```python
from build123d import *

# Parameters (mm, degrees)
SKETCH_1_R               = 72.2
EXTRUDE_1_DEPTH          = 9
CUT_EXTRUDE_START        = -9
CUT_EXTRUDE_2_DEPTH      = 9
SKETCH_3_R               = 47
CUT_EXTRUDE_3_DEPTH      = 3
CUT_EXTRUDE_START_2      = -3
SKETCH_4_R               = 47
CUT_EXTRUDE_4_DEPTH      = 3
SKETCH_6_R               = 2
CUT_EXTRUDE_6_DEPTH      = 3
PATTERN_CIRCULAR_1_COUNT = 14
SKETCH_5_R               = 13
SKETCH_5_R_2             = 2.5
SKETCH_5_R_3             = 10.5
CUT_EXTRUDE_7_DEPTH      = 102.792337629


with BuildPart() as part:
    # 草图1 → 凸台-拉伸1 (new body)
    with BuildSketch(Plane.XY):
        Circle(SKETCH_1_R)
    extrude(amount=EXTRUDE_1_DEPTH)

    # 草图2 → 切除-拉伸2 (cut)
    with BuildSketch(Plane.XY.offset(9).offset(CUT_EXTRUDE_START)):
        with BuildLine():
            Line((-10, 71.504125755), (-10, 59.666070761))
            ThreePointArc((-10, 59.666070761), (-9.316897592, 58.160819708), (-7.734219269, 57.683809273))
            ThreePointArc((-7.734219269, 57.683809273), (0, 58.2), (7.734219269, 57.683809273))
            ThreePointArc((7.734219269, 57.683809273), (9.316897592, 58.160819708), (10, 59.666070761))
            Line((10, 59.666070761), (10, 71.504125755))
            ThreePointArc((10, 71.504125755), (0, 72.2), (-10, 71.504125755))
        make_face()
        with BuildLine():
            Line((22.014788766, 68.761828623), (16.878449201, 58.096109616))
            ThreePointArc((16.878449201, 58.096109616), (16.840799249, 56.443538253), (18.059776075, 55.327068313))
            ThreePointArc((18.059776075, 55.327068313), (25.252033617, 52.436388112), (31.996357633, 48.615564362))
            ThreePointArc((31.996357633, 48.615564362), (33.629268601, 48.358637524), (34.897826559, 49.418434834))
            Line((34.897826559, 49.418434834), (40.034166124, 60.084153841))
            ThreePointArc((40.034166124, 60.084153841), (31.326405964, 65.049952263), (22.014788766, 68.761828623))
        make_face()
        with BuildLine():
            Line((49.669278623, 52.400408024), (40.413914537, 45.019501461))
            ThreePointArc((40.413914537, 45.019501461), (39.66296926, 43.546921812), (40.276811279, 42.012122931))
            ThreePointArc((40.276811279, 42.012122931), (45.50259228, 36.287106468), (49.921224958, 29.918410697))
            ThreePointArc((49.921224958, 29.918410697), (51.280950528, 28.978434099), (52.883710574, 29.382871811))
            Line((52.883710574, 29.382871811), (62.13907466, 36.763778374))
            ThreePointArc((62.13907466, 36.763778374), (56.448233034, 45.015963694), (49.669278623, 52.400408024))
        make_face()
        with BuildLine():
            Line((67.486158695, 25.660443967), (55.944908455, 23.026228913))
            ThreePointArc((55.944908455, 23.026228913), (54.629401775, 22.025303439), (54.516530046, 20.376161358))
            ThreePointArc((54.516530046, 20.376161358), (56.740804489, 12.950718356), (57.958581437, 5.295548869))
            ThreePointArc((57.958581437, 5.295548869), (58.775811283, 3.858696403), (60.395327134, 3.527670669))
            Line((60.395327134, 3.527670669), (71.936577374, 6.161885723))
            ThreePointArc((71.936577374, 6.161885723), (70.38979526, 16.066011432), (67.486158695, 25.660443967))
        make_face()
        with BuildLine():
            Line((71.936577374, -6.161885723), (60.395327134, -3.527670669))
            ThreePointArc((60.395327134, -3.527670669), (58.775811283, -3.858696403), (57.958581437, -5.295548869))
            ThreePointArc((57.958581437, -5.295548869), (56.740804489, -12.950718356), (54.516530046, -20.376161358))
            ThreePointArc((54.516530046, -20.376161358), (54.629401775, -22.025303439), (55.944908455, -23.026228913))
            Line((55.944908455, -23.026228913), (67.486158695, -25.660443967))
            ThreePointArc((67.486158695, -25.660443967), (70.38979526, -16.066011432), (71.936577374, -6.161885723))
        make_face()
        with BuildLine():
            Line((62.13907466, -36.763778374), (52.883710574, -29.382871811))
            ThreePointArc((52.883710574, -29.382871811), (51.280950528, -28.978434099), (49.921224958, -29.918410697))
            ThreePointArc((49.921224958, -29.918410697), (45.50259228, -36.287106468), (40.276811279, -42.012122931))
            ThreePointArc((40.276811279, -42.012122931), (39.66296926, -43.546921812), (40.413914537, -45.019501461))
            Line((40.413914537, -45.019501461), (49.669278623, -52.400408024))
            ThreePointArc((49.669278623, -52.400408024), (56.448233034, -45.015963694), (62.13907466, -36.763778374))
        make_face()
        with BuildLine():
            Line((40.034166124, -60.084153841), (34.897826559, -49.418434834))
            ThreePointArc((34.897826559, -49.418434834), (33.629268601, -48.358637524), (31.996357633, -48.615564362))
            ThreePointArc((31.996357633, -48.615564362), (25.252033617, -52.436388112), (18.059776075, -55.327068313))
            ThreePointArc((18.059776075, -55.327068313), (16.840799249, -56.443538253), (16.878449201, -58.096109616))
            Line((16.878449201, -58.096109616), (22.014788766, -68.761828623))
            ThreePointArc((22.014788766, -68.761828623), (31.326405964, -65.049952263), (40.034166124, -60.084153841))
        make_face()
        with BuildLine():
            Line((10, -71.504125755), (10, -59.666070761))
            ThreePointArc((10, -59.666070761), (9.316897592, -58.160819708), (7.734219269, -57.683809273))
            ThreePointArc((7.734219269, -57.683809273), (0, -58.2), (-7.734219269, -57.683809273))
            ThreePointArc((-7.734219269, -57.683809273), (-9.316897592, -58.160819708), (-10, -59.666070761))
            Line((-10, -59.666070761), (-10, -71.504125755))
            ThreePointArc((-10, -71.504125755), (0, -72.2), (10, -71.504125755))
        make_face()
        with BuildLine():
            Line((-22.014788766, -68.761828623), (-16.878449201, -58.096109616))
            ThreePointArc((-16.878449201, -58.096109616), (-16.840799249, -56.443538253), (-18.059776075, -55.327068313))
            ThreePointArc((-18.059776075, -55.327068313), (-25.252033617, -52.436388112), (-31.996357633, -48.615564362))
            ThreePointArc((-31.996357633, -48.615564362), (-33.629268601, -48.358637524), (-34.897826559, -49.418434834))
            Line((-34.897826559, -49.418434834), (-40.034166124, -60.084153841))
            ThreePointArc((-40.034166124, -60.084153841), (-31.326405964, -65.049952263), (-22.014788766, -68.761828623))
        make_face()
        with BuildLine():
            Line((-49.669278623, -52.400408024), (-40.413914537, -45.019501461))
            ThreePointArc((-40.413914537, -45.019501461), (-39.66296926, -43.546921812), (-40.276811279, -42.012122931))
            ThreePointArc((-40.276811279, -42.012122931), (-45.50259228, -36.287106468), (-49.921224958, -29.918410697))
            ThreePointArc((-49.921224958, -29.918410697), (-51.280950528, -28.978434099), (-52.883710574, -29.382871811))
            Line((-52.883710574, -29.382871811), (-62.13907466, -36.763778374))
            ThreePointArc((-62.13907466, -36.763778374), (-56.448233034, -45.015963694), (-49.669278623, -52.400408024))
        make_face()
        with BuildLine():
            Line((-67.486158695, -25.660443967), (-55.944908455, -23.026228913))
            ThreePointArc((-55.944908455, -23.026228913), (-54.629401775, -22.025303439), (-54.516530046, -20.376161358))
            ThreePointArc((-54.516530046, -20.376161358), (-56.740804489, -12.950718356), (-57.958581437, -5.295548869))
            ThreePointArc((-57.958581437, -5.295548869), (-58.775811283, -3.858696403), (-60.395327134, -3.527670669))
            Line((-60.395327134, -3.527670669), (-71.936577374, -6.161885723))
            ThreePointArc((-71.936577374, -6.161885723), (-70.38979526, -16.066011432), (-67.486158695, -25.660443967))
        make_face()
        with BuildLine():
            Line((-71.936577374, 6.161885723), (-60.395327134, 3.527670669))
            ThreePointArc((-60.395327134, 3.527670669), (-58.775811283, 3.858696403), (-57.958581437, 5.295548869))
            ThreePointArc((-57.958581437, 5.295548869), (-56.740804489, 12.950718356), (-54.516530046, 20.376161358))
            ThreePointArc((-54.516530046, 20.376161358), (-54.629401775, 22.025303439), (-55.944908455, 23.026228913))
            Line((-55.944908455, 23.026228913), (-67.486158695, 25.660443967))
            ThreePointArc((-67.486158695, 25.660443967), (-70.38979526, 16.066011432), (-71.936577374, 6.161885723))
        make_face()
        with BuildLine():
            Line((-62.13907466, 36.763778374), (-52.883710574, 29.382871811))
            ThreePointArc((-52.883710574, 29.382871811), (-51.280950528, 28.978434099), (-49.921224958, 29.918410697))
            ThreePointArc((-49.921224958, 29.918410697), (-45.50259228, 36.287106468), (-40.276811279, 42.012122931))
            ThreePointArc((-40.276811279, 42.012122931), (-39.66296926, 43.546921812), (-40.413914537, 45.019501461))
            Line((-40.413914537, 45.019501461), (-49.669278623, 52.400408024))
            ThreePointArc((-49.669278623, 52.400408024), (-56.448233034, 45.015963694), (-62.13907466, 36.763778374))
        make_face()
        with BuildLine():
            Line((-40.034166124, 60.084153841), (-34.897826559, 49.418434834))
            ThreePointArc((-34.897826559, 49.418434834), (-33.629268601, 48.358637524), (-31.996357633, 48.615564362))
            ThreePointArc((-31.996357633, 48.615564362), (-25.252033617, 52.436388112), (-18.059776075, 55.327068313))
            ThreePointArc((-18.059776075, 55.327068313), (-16.840799249, 56.443538253), (-16.878449201, 58.096109616))
            Line((-16.878449201, 58.096109616), (-22.014788766, 68.761828623))
            ThreePointArc((-22.014788766, 68.761828623), (-31.326405964, 65.049952263), (-40.034166124, 60.084153841))
        make_face()
    extrude(amount=CUT_EXTRUDE_2_DEPTH, mode=Mode.SUBTRACT)

    # 草图3 → 切除-拉伸3 (cut)
    with BuildSketch(Plane.XY.offset(9)):
        Circle(SKETCH_3_R)
    extrude(amount=-CUT_EXTRUDE_3_DEPTH, mode=Mode.SUBTRACT)

    # 草图4 → 切除-拉伸4 (cut)
    with BuildSketch(Plane(origin=(0, 0, 0), x_dir=(-1, 0, 0), z_dir=(0, 0, -1)).offset(CUT_EXTRUDE_START_2)):
        with Locations(Location((0, 0, 0), (0, 0, 180))):
            Circle(SKETCH_4_R)
    extrude(amount=CUT_EXTRUDE_4_DEPTH, mode=Mode.SUBTRACT)

    # 草图6 → 切除-拉伸6 (cut)
    with BuildSketch(Plane(origin=(-10, 0, 0), x_dir=(0, 0, -1), z_dir=(1, 0, 0))):
        with Locations((-4.5, 66.154125755)):
            Circle(SKETCH_6_R)
    cut_extrude_6 = extrude(amount=-CUT_EXTRUDE_6_DEPTH, mode=Mode.SUBTRACT)

    # 阵列(圆周)1: 切除-拉伸6 ×14 about axis
    pattern_circular_1_axis = Axis((0, 0, 0), (0, 0, 1))
    for i in range(1, PATTERN_CIRCULAR_1_COUNT):
        add(cut_extrude_6.rotate(pattern_circular_1_axis, i * 360 / PATTERN_CIRCULAR_1_COUNT), mode=Mode.SUBTRACT)

    # 草图5 → 切除-拉伸7 (cut, through all)
    with BuildSketch(Plane(origin=(0, 0, 3), x_dir=(-1, 0, 0), z_dir=(0, 0, -1))):
        Circle(SKETCH_5_R)
        with Locations((-6.479848807, 22.068338393)):
            Circle(SKETCH_5_R_2)
        with Locations((15.871817264, 16.645882876)):
            Circle(SKETCH_5_R_2)
        with Locations((22.351666071, -5.422455517)):
            Circle(SKETCH_5_R_2)
        with Locations((6.479848807, -22.068338393)):
            Circle(SKETCH_5_R_2)
        with Locations((-15.871817264, -16.645882876)):
            Circle(SKETCH_5_R_2)
        with Locations((-22.351666071, 5.422455517)):
            Circle(SKETCH_5_R_2)
        with Locations((8.251562743, 34.013404891)):
            Circle(SKETCH_5_R_3)
        with Locations((33.582254077, 9.860639489)):
            Circle(SKETCH_5_R_3)
        with Locations((25.330691334, -24.152765402)):
            Circle(SKETCH_5_R_3)
        with Locations((-8.251562743, -34.013404891)):
            Circle(SKETCH_5_R_3)
        with Locations((-33.582254077, -9.860639489)):
            Circle(SKETCH_5_R_3)
        with Locations((-25.330691334, 24.152765402)):
            Circle(SKETCH_5_R_3)
    extrude(amount=-CUT_EXTRUDE_7_DEPTH, mode=Mode.SUBTRACT)


solid = part.part
```
Source: CAD feature listing. Evaluate the final solid. Frame: model axes, mm. A direction names the side the tool comes from. Round coordinates to 2 decimals unless told otherwise and drop trailing zeros. Order: outer loops, then holes, each group sorted by start corner. A loop starts at its lowest first (then second) coordinate and runs counter-clockwise, first axis right, second up. Notation, with made-up numbers: (24, 87) -> (74, 87) arc R30 cw to (74, 125) -> close; hole circle Ø6 at (-14.5, 82). An arc over 180 degrees is marked (long way). One line per item, written item: value. Start each with the question number.
Q1. Access query for faces 5 (the flat face through (-36.93, 53.64, 2.44)), 6 (the flat face through (-44.98, 48.66, 4.44)), 7 (the flat face through (40.43, -53.99, 4.53)), 8 (the cylindrical face through (-45.57, 36.2, 4.44)). Directions: +Z, -Z, +X, -X, +Y, -Y. A direction counts if a zero-diameter tool reaches every point of the face in a straight line with its end or side. Return the directions, or none.
Q2. Draft query along Z for faces 1 (the flat face through (67.416, -2.053, 4.528)), 2 (the cylindrical face through (-11.479, 67.841, 3.425)), 3 (the flat face through (-43, -21, 0)), 4 (the cylindrical face through (0.1, -58.2, 4.4)). Return one class per face: pulls with the +Z half, pulls with the -Z half, needs draft (parallel to the pull), parting line crosses it, or undercut.
Q3. Section query A-A (x = 0). Return the cut outline in (y, z).
Q4. Pin query (flat end, axial travel): pin 1 (4.5 mm diameter, centred on x = -22.35, y = -5.42, fed in from +Z); pin 2 (1.5 mm diameter, centred on x = -45, z = 5, fed in from +Y); pin 3 (2.5 mm diameter, centred on y = 65, z = 3, fed in from +X); pin 4 (2 mm diameter, centred on y = 18, z = 7.5, fed in from -X). Return the tip coordinate at first contact, or that it passes through.
Q5. Section query B-B (z = 4.5). Give the number of separate pieces and of enclosed holes in the cut face, plus the area to 3 significant figures.
Q6. Material intervals for probe 1 along Y at (x, z) = (35, 3.25); probe 2 along X at (y, z) = (-48.5, 0.5); probe 3 along Y at (x, z) = (48, 8.25), sorted ascending.
Findings below:
1. face 5: +Z, -Z, +Y
1. face 6: +Z, -Z, -X
1. face 7: none
1. face 8: +Z, -Z
2. face 1: undercut
2. face 2: undercut
2. face 3: pulls with the -Z half
2. face 4: needs draft
3. outline: (-58.2, 0) -> (-47, 0) -> (-47, 3) -> (-40.51, 3) -> (-40.51, 6) -> (-47, 6) -> (-47, 9) -> (-58.2, 9) -> close; (-27.52, 3) -> (-13, 3) -> (-13, 6) -> (-27.52, 6) -> close; (13, 3) -> (27.52, 3) -> (27.52, 6) -> (13, 6) -> close; (40.51, 3) -> (47, 3) -> (47, 0) -> (58.2, 0) -> (58.2, 9) -> (47, 9) -> (47, 6) -> (40.51, 6) -> close
4. pin 1: through
4. pin 2: y = 57.05
4. pin 3: x = 20.81
4. pin 4: x = -55.66
5. separate pieces: 1
5. enclosed holes: 13
5. area: 9,580 mm²
6. probe 1: -49.63 to -20.26, 0.54 to 20.06, 28.25 to 49.63
6. probe 2: -44.78 to -34, -32.2 to 32.2, 34 to 44.78
6. probe 3: -53.93 to -51.07, -32.91 to 32.91, 51.07 to 53.93
